Geometry: final body of the model. Coordinates: model frame, mm. A direction names the side the tool comes from. Coordinates: 2 decimals unless noted, no trailing zeros. Write each loop counter-clockwise with the first axis right and the second up, starting at its lowest first coordinate (ties: lowest second). Pieces come first, ordered by that corner, then holes. Notation, with made-up numbers: (-23.5, 5.5) - (31.5, 5.5) arc R23 cw to (31.5, 14.5) - close; hole circle Ø11 at (-35.75, 32.25). An arc over 180 degrees is marked (long way). Answer as a JSON object with one key per item and string values. Group by question number.
Item 1: First-contact query: pin 1 Ø1.1 at (y, z) = (-6.5, -4.5) entering from -X; pin 2 Ø6 at (x, y) = (-1.5, -1) entering from +Z; pin 3 Ø1 at (y, z) = (-1, -4.5) entering from -X; pin 4 Ø2 at (y, z) = (7, -3.5) entering from -X. Flat tips, straight axial feed; report the tip coordinate or a pass-through.
Item 2: Section C-C on z = -3. Return loops of the section in (x, y).
Item 3: Mould query, pull axis Y, two halves, no side actions, for faces 4 (the flat face through (5.657, 7, -4)), 5 (the cylindrical face through (-5.66, -0.12, -3.63)), 6 (the cylindrical face through (25.57, 7.05, -4.27)), 7 (the flat face through (18, -5.66, -5)). Classes: pulls with the +Y half, pulls with the -Y half, needs draft (parallel to the pull), parting line crosses it, or undercut.
Item 4: Section D-D on y = -1.5. Return loops of the section in (x, z), and give its area (3 significant figures).
Item 5: Section A-A on x = 12. Return loops of the section in (y, z).
Item 6: Section B-B on y = 0. Return loops of the section in (x, z), and give its area (3 significant figures).
Item 7: Set-up query: faces 1 (the flat face through (9, -6, -4)), 2 (the cylindrical face through (14.5, 0.1, -5.4)), 3 (the flat face through (16, 5.657, -5)). Return all of +Z, -Z, +X, -X, +Y, -Y with unobstructed straight access to the full face (end or side cutting, diameter ignored); none if empty.
Item 8: Line query: line 1 along Y through (x, z) = (18, -4.9); line 2 along Y through (x, z) = (0, -4.2); line 3 along Y through (x, z) = (12, -3.4). Output: solid intervals per line, ascending. Write a range as from..to.
```python
from build123d import *

# Parameters (mm, degrees)
BOSS_EXTRUDE1_DEPTH = 2
BOSS_EXTRUDE2_START = 2.5
BOSS_EXTRUDE2_DEPTH = 2.5
CUT_EXTRUDE1_DEPTH  = 2.5
BOSS_EXTRUDE3_DEPTH = 2.3
SKETCH9_R           = 2.1
CUT_EXTRUDE2_DEPTH  = 2.5
SKETCH10_R          = 2.5
BOSS_EXTRUDE4_DEPTH = 1.2
SKETCH11_R          = 0.95
CUT_EXTRUDE3_DEPTH  = 9.2
SKETCH12_R          = 2
CUT_EXTRUDE4_DEPTH  = 2.5
SKETCH14_W          = 20.343145751
SKETCH14_H          = 1.841510486
SKETCH14_W_2        = 17
SKETCH14_H_2        = 1.34163614
BOSS_EXTRUDE5_DEPTH = 1.2
FILLET1_R           = 1.5
SKETCH17_R          = 0.95
CUT_EXTRUDE5_DEPTH  = 3


# Read off the part's stored shape, not the designer's step: Boss-Extrude3
with BuildPart() as part:
    # Sketch5 → Boss-Extrude1 (new body)
    with BuildSketch(Plane.XY):
        with BuildLine():
            Line((8, 0), (9, -2.501635265))
            Line((9, -2.501635265), (9, -7.001635265))
            Line((9, -7.001635265), (26, -7.001635265))
            Line((26, -7.001635265), (26, 7.498364735))
            Line((26, 7.498364735), (5.656854249, 7.498364735))
            Line((5.656854249, 7.498364735), (5.656854249, 5.656854249))
            ThreePointArc((5.656854249, 5.656854249), (7.39103626, 3.061467459), (8, 0))
        make_face()
    extrude(amount=BOSS_EXTRUDE1_DEPTH)

    # Sketch6 → Boss-Extrude2 (add)
    with BuildSketch(Plane(origin=(0, 0, 0), x_dir=(-1, 0, 0), z_dir=(0, 0, -1)).offset(BOSS_EXTRUDE2_START)):
        with BuildLine():
            Line((-5.656854249, 7.498364735), (-5.656854249, 5.656854249))
            ThreePointArc((-5.656854249, 5.656854249), (-7.39103626, 3.061467459), (-8, 0))
            Line((-8, 0), (-9, -2.501635265))
            Line((-9, -2.501635265), (-9, -7.001635265))
            Line((-9, -7.001635265), (-26, -7.001635265))
            Line((-26, -7.001635265), (-26, 7.498364735))
            Line((-26, 7.498364735), (-5.656854249, 7.498364735))
        make_face()
    extrude(amount=-BOSS_EXTRUDE2_DEPTH)

    # Sketch7 → Cut-Extrude1 (cut)
    with BuildSketch(Plane(origin=(0, 0, -2.5), x_dir=(-1, 0, 0), z_dir=(0, 0, -1))):
        Polygon((-26, 5.298364735), (-2.738141148, 5.298364735), (-2.738141148, 3.998364735), (-29.849535112, 3.998364735), (-29.849535112, 5.298364735), align=None)
    extrude(amount=-CUT_EXTRUDE1_DEPTH, mode=Mode.SUBTRACT)

    # Boss-Extrude3 outline → Boss-Extrude3 (add)
    with BuildSketch(Plane(origin=(0, 0, -2.5), x_dir=(-1, 0, 0), z_dir=(0, 0, -1))):
        with BuildLine():
            Line((-9, -7.001635265), (-9, -5.659999125))
            Line((-9, -5.659999125), (0, -5.659998688))
            ThreePointArc((0, -5.659998688), (5.659998688, 0), (0, 5.659998688))
            Line((0, 5.659998688), (-5.656854249, 5.656854249))
            Line((-5.656854249, 5.656854249), (-5.656854249, 7.498364735))
            Line((-5.656854249, 7.498364735), (-26, 7.498364735))
            Line((-26, 7.498364735), (-26, -7.001635265))
            Line((-26, -7.001635265), (-9, -7.001635265))
        make_face()
    extrude(amount=BOSS_EXTRUDE3_DEPTH)

    # Sketch9 → Cut-Extrude2 (cut)
    with BuildSketch(Plane(origin=(0, 0, -4.8), x_dir=(-1, 0, 0), z_dir=(0, 0, -1))):
        Circle(SKETCH9_R)
    extrude(amount=-CUT_EXTRUDE2_DEPTH, mode=Mode.SUBTRACT)

    # Sketch10 → Boss-Extrude4 (add)
    with BuildSketch(Plane(origin=(0, 0, -4.8), x_dir=(-1, 0, 0), z_dir=(0, 0, -1))):
        with Locations((-12, 0)):
            Circle(SKETCH10_R)
        with Locations((-18, 0)):
            Circle(SKETCH10_R)
    extrude(amount=BOSS_EXTRUDE4_DEPTH)

    # Sketch11 → Cut-Extrude3 (cut)
    with BuildSketch(Plane(origin=(0, 0, -6), x_dir=(-1, 0, 0), z_dir=(0, 0, -1))):
        with Locations((-18, 0)):
            Circle(SKETCH11_R)
        with Locations((-12, 0)):
            Circle(SKETCH11_R)
    extrude(amount=-CUT_EXTRUDE3_DEPTH, mode=Mode.SUBTRACT)

    # Sketch12 → Cut-Extrude4 (cut)
    with BuildSketch(Plane.XY.offset(2)):
        with Locations((12, 0)):
            Circle(SKETCH12_R)
        with Locations((18, 0)):
            Circle(SKETCH12_R)
    extrude(amount=-CUT_EXTRUDE4_DEPTH, mode=Mode.SUBTRACT)

    # Sketch14 → Boss-Extrude5 (add)
    with BuildSketch(Plane(origin=(0, 0, -4.8), x_dir=(-1, 0, 0), z_dir=(0, 0, -1))):
        with Locations((-15.828427124, 6.577609492)):
            Rectangle(SKETCH14_W, SKETCH14_H)
        with Locations((-17.5, -6.330817195)):
            Rectangle(SKETCH14_W_2, SKETCH14_H_2)
    extrude(amount=BOSS_EXTRUDE5_DEPTH)

    # Fillet1
    # the kernel refuses this fillet: 1.5 mm, written as the material it takes off along each edge
    with BuildSketch(Plane(origin=(24.5, -5.501635265, 0.5), x_dir=(0, 0, 1), z_dir=(0, -1, 0))) as fillet1_piece_1_section:
        Polygon((0, 0), (FILLET1_R, 0), (FILLET1_R, -FILLET1_R), (0, -FILLET1_R), align=None)
    fillet1_piece_1 = extrude(amount=FILLET1_R, mode=Mode.PRIVATE)
    fillet1_piece_1 = fillet1_piece_1 - Plane(origin=(24.5, -5.501635265, 0.5), x_dir=(-0.7071067811865475, 0, -0.7071067811865475), z_dir=(0, -1, 0)) * Sphere(FILLET1_R, mode=Mode.PRIVATE)
    add(fillet1_piece_1, mode=Mode.SUBTRACT)
    with BuildSketch(Plane(origin=(24.5, 5.998364735, 0.5), x_dir=(0, 0, 1), z_dir=(0, 1, 0))) as fillet1_piece_2_section:
        Polygon((0, 0), (FILLET1_R, 0), (FILLET1_R, FILLET1_R), (0, FILLET1_R), align=None)
    fillet1_piece_2 = extrude(amount=FILLET1_R, mode=Mode.PRIVATE)
    fillet1_piece_2 = fillet1_piece_2 - Plane(origin=(24.5, 5.998364735, 0.5), x_dir=(-0.7071067811865475, 0, -0.7071067811865475), z_dir=(0, 1, 0)) * Sphere(FILLET1_R, mode=Mode.PRIVATE)
    add(fillet1_piece_2, mode=Mode.SUBTRACT)
    with BuildSketch(Plane(origin=(26, -5.501635265, 2), x_dir=(-1, 0, 0), z_dir=(0, 1, 0))) as fillet1_piece_3:
        with BuildLine():
            CenterArc((FILLET1_R, -FILLET1_R), FILLET1_R, 90, 90)
            Line((0, -FILLET1_R), (0, 0))
            Line((0, 0), (FILLET1_R, 0))
        make_face()
    extrude(amount=11.5, mode=Mode.SUBTRACT)
    with BuildSketch(Plane(origin=(26, -7.001635265, -2.5), x_dir=(-1, 0, 0), z_dir=(0, 0, 1))) as fillet1_piece_4:
        with BuildLine():
            CenterArc((FILLET1_R, -FILLET1_R), FILLET1_R, 90, 90)
            Line((0, -FILLET1_R), (0, 0))
            Line((0, 0), (FILLET1_R, 0))
        make_face()
    extrude(amount=3, mode=Mode.SUBTRACT)
    with BuildSketch(Plane(origin=(5.25, -7.001635265, 2), x_dir=(0, 1, 0), z_dir=(1, 0, 0))) as fillet1_piece_5:
        with BuildLine():
            CenterArc((FILLET1_R, -FILLET1_R), FILLET1_R, 90, 90)
            Line((0, -FILLET1_R), (0, 0))
            Line((0, 0), (FILLET1_R, 0))
        make_face()
    extrude(amount=19.25, mode=Mode.SUBTRACT)
    with BuildSketch(Plane(origin=(24.5, 7.498364735, 2), x_dir=(0, -1, 0), z_dir=(-1, 0, 0))) as fillet1_piece_6:
        with BuildLine():
            CenterArc((FILLET1_R, -FILLET1_R), FILLET1_R, 90, 90)
            Line((0, -FILLET1_R), (0, 0))
            Line((0, 0), (FILLET1_R, 0))
        make_face()
    extrude(amount=22.593145751, mode=Mode.SUBTRACT)
    with BuildSketch(Plane(origin=(26, 7.498364735, -2.5), x_dir=(-1, 0, 0), z_dir=(0, 0, 1))) as fillet1_piece_7:
        with BuildLine():
            CenterArc((FILLET1_R, FILLET1_R), FILLET1_R, 180, 90)
            Line((0, FILLET1_R), (0, 0))
            Line((0, 0), (FILLET1_R, 0))
        make_face()
    extrude(amount=3, mode=Mode.SUBTRACT)
    with BuildSketch(Plane(origin=(26, 7.498364735, -2.5), x_dir=(-1.0, -1.9174232572065026e-10, 0), z_dir=(0, 0, -1))) as fillet1_piece_8:
        with BuildLine():
            CenterArc((FILLET1_R, -FILLET1_R), FILLET1_R, 90.000000011, 90)
            Line((FILLET1_R * 1.9173522033e-10, -FILLET1_R), (0, 0))
            Line((0, 0), (FILLET1_R, 0))
        make_face()
    extrude(amount=2.3, mode=Mode.SUBTRACT)
    with BuildSketch(Plane(origin=(26, 7.498364735, -4.8), x_dir=(-1, 0, 0), z_dir=(0, 0, -1))) as fillet1_piece_9:
        with BuildLine():
            CenterArc((FILLET1_R, -FILLET1_R), FILLET1_R, 90, 90)
            Line((0, -FILLET1_R), (0, 0))
            Line((0, 0), (FILLET1_R, 0))
        make_face()
    extrude(amount=4.95, mode=Mode.SUBTRACT)
    with BuildSketch(Plane(origin=(26, -7.001635265, -2.5), x_dir=(-1.0, -1.9169850891861218e-10, 0), z_dir=(0, 0, -1))) as fillet1_piece_10:
        with BuildLine():
            CenterArc((FILLET1_R, FILLET1_R), FILLET1_R, 180.000000011, 90)
            Line((-FILLET1_R * 1.91707982785e-10, FILLET1_R), (0, 0))
            Line((0, 0), (FILLET1_R, 0))
        make_face()
    extrude(amount=2.3, mode=Mode.SUBTRACT)
    with BuildSketch(Plane(origin=(26, -7.001635265, -4.8), x_dir=(-1, 0, 0), z_dir=(0, 0, -1))) as fillet1_piece_11:
        with BuildLine():
            CenterArc((FILLET1_R, FILLET1_R), FILLET1_R, 180, 90)
            Line((0, FILLET1_R), (0, 0))
            Line((0, 0), (FILLET1_R, 0))
        make_face()
    extrude(amount=4.95, mode=Mode.SUBTRACT)

    # Sketch17 → Cut-Extrude5 (cut)
    with BuildSketch(Plane.XZ.offset(7.001635265)):
        with Locations((22, -1)):
            Circle(SKETCH17_R)
        with Locations((18, -1)):
            Circle(SKETCH17_R)
    extrude(amount=-CUT_EXTRUDE5_DEPTH, mode=Mode.SUBTRACT)


with BuildPart() as body_2:
    # Split1: the piece on the far side of the plane
    add(part.part)
    split(bisect_by=Plane(origin=(0, 0, -2.5), x_dir=(-1, 0, 0), z_dir=(0, 0, -1)), keep=Keep.BOTTOM)


with BuildPart() as part_1:
    add(part.part)

    # Split1
    split(bisect_by=Plane(origin=(0, 0, -2.5), x_dir=(-1, 0, 0), z_dir=(0, 0, -1)), keep=Keep.TOP)


solid = part_1.part
```
Checks:
{
 "1": {"pin 1": "x = 9", "pin 2": "z = -2.5", "pin 3": "x = -5.64", "pin 4": "x = 5.66"},
 "2": {"outline": "(0, -5.66) - (9, -5.66) - (9, -7) - (24.5, -7) arc R1.5 ccw to (26, -5.5) - (26, 6) arc R1.5 ccw to (24.5, 7.5) - (5.66, 7.5) - (5.66, 5.66) - (0, 5.66) arc R5.66 ccw to start; hole circle Ø4.2 at (0, 0); hole circle Ø1.9 at (12, 0); hole circle Ø1.9 at (18, 0)"},
 "3": {"face 4": "needs draft", "face 5": "parting line crosses it", "face 6": "pulls with the +Y half", "face 7": "undercut"},
 "4": {"outline": "(-5.46, -4.8) - (-1.47, -4.8) - (-1.47, -2.5) - (-5.46, -2.5) - close; (1.47, -4.8) - (10, -4.8) - (10, -6) - (14, -6) - (14, -4.8) - (16, -4.8) - (16, -6) - (20, -6) - (20, -4.8) - (26, -4.8) - (26, -2.5) - (1.47, -2.5) - close", "area": "75.2 mm^2"},
 "5": {"outline": "(-7, -6) - (-5.66, -6) - (-5.66, -4.8) - (-2.5, -4.8) - (-2.5, -6) - (-0.95, -6) - (-0.95, -2.5) - (-7, -2.5) - close; (0.95, -6) - (2.5, -6) - (2.5, -4.8) - (5.66, -4.8) - (5.66, -6) - (7.5, -6) - (7.5, -2.5) - (0.95, -2.5) - close"},
 "6": {"outline": "(-5.66, -4.8) - (-2.1, -4.8) - (-2.1, -2.5) - (-5.66, -2.5) - close; (2.1, -4.8) - (9.5, -4.8) - (9.5, -6) - (11.05, -6) - (11.05, -2.5) - (2.1, -2.5) - close; (12.95, -6) - (14.5, -6) - (14.5, -4.8) - (15.5, -4.8) - (15.5, -6) - (17.05, -6) - (17.05, -2.5) - (12.95, -2.5) - close; (18.95, -6) - (20.5, -6) - (20.5, -4.8) - (26, -4.8) - (26, -2.5) - (18.95, -2.5) - close", "area": "61.9 mm^2"},
 "7": {"face 1": "+Z, -Z, -X, -Y", "face 2": "-Z", "face 3": "-Z, +X, -X"},
 "8": {"line 1": "-7..-5.66, -2.5..-0.95, 0.95..2.5, 5.66..7.5", "line 2": "-5.66..-2.1, 2.1..5.66", "line 3": "-7..-0.95, 0.95..7.5"}
}
